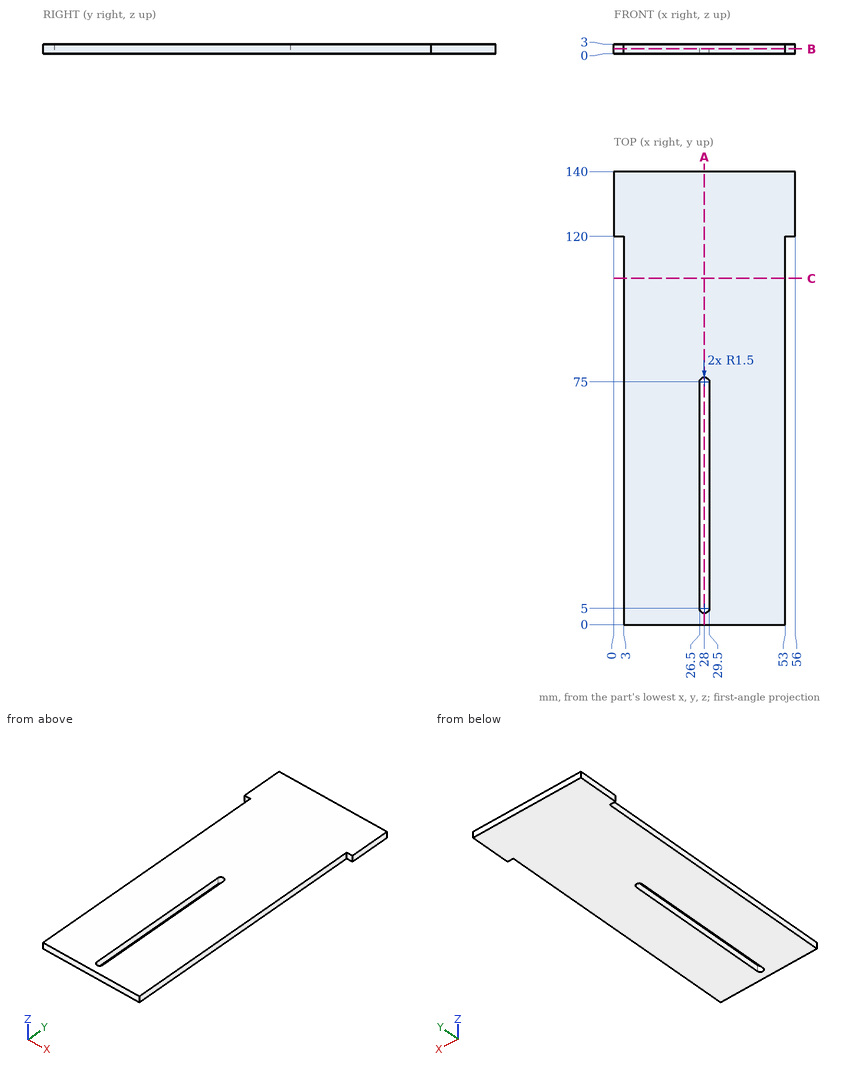
Source: three-view drawing plus pictorial views. Frame: mm from the lowest corner of the part. Round coordinates to 2 decimals unless told otherwise and drop trailing zeros. Loops run counter-clockwise (first coordinate to the right, second up) from the corner with the lowest first, then second, coordinate; pieces in that order, holes last. Notation, with made-up numbers: M 54,2 L 79,2 A8 ccw 79,15 Z; hole C 84,60.5 d2. An arc over 180 degrees is marked long. Answer as CSV lines item,"result". Start each with the question number.
(1) Section A-A, the plane x = 28. Output: boundary loops of the cut face in (y, z), plus the area to 3 significant figures.
(2) Line query: line 1 (X direction, y = 41.5, z = 2.35); line 2 (X direction, y = 115, z = 0.3); line 3 (Y direction, x = 28.5, z = 0.7). Output: solid intervals per line, ascending. Write a range as [from, to].
(3) Section B-B, the plane z = 1.5. Output: boundary loops of the cut face in (x, y), plus the area to 3 significant figures.
(4) Section C-C, the plane y = 107. Output: boundary loops of the cut face in (x, z), plus the area to 3 significant figures.
(5) First-contact query: pin 1 (4 mm diameter, centred on x = 23.5, y = 106.5, fed in from -Z); pin 2 (1.5 mm diameter, centred on y = 30, z = 2, fed in from -X); pin 3 (1.5 mm diameter, centred on x = 54, z = 1, fed in from -Y). Flat tips, straight axial feed; report the tip coordinate or a pass-through.
Values found:
1,outline,"M 0,0 L 3.5,0 L 3.5,3 L 0,3 Z; M 76.5,0 L 140,0 L 140,3 L 76.5,3 Z"
1,area,"201 mm²"
2,line 1,"x = [3, 26.5], [29.5, 53]"
2,line 2,"x = [3, 53]"
2,line 3,"y = [0, 3.59], [76.41, 140]"
3,outline,"M 0,120 L 3,120 L 3,0 L 53,0 L 53,120 L 56,120 L 56,140 L 0,140 Z; hole M 26.5,5 A1.5 ccw 29.5,5 L 29.5,75 A1.5 ccw 26.5,75 Z"
3,area,"6,900 mm²"
4,outline,"M 3,0 L 53,0 L 53,3 L 3,3 Z"
4,area,"150 mm²"
5,pin 1,"stops at z = 0"
5,pin 2,"stops at x = 3"
5,pin 3,"stops at y = 120"
